```python
from build123d import *

# Parameters (mm, degrees)
SKETCH_1_W          = 30
SKETCH_1_H          = 16
EXTRUDE_1_DEPTH     = 2
EXTRUDE_2_DEPTH     = 1
SKETCH_3_R          = 2.5
EXTRUDE_3_DEPTH     = 15
SKETCH_4_W          = 7.5
SKETCH_4_H          = 13
SKETCH_5_R          = 3
CUT_EXTRUDE_1_DEPTH = 27.248809497


with BuildPart() as part:
    # 草圖1 → 填料-伸長1 (new body)
    with BuildSketch(Plane.XY):
        Rectangle(SKETCH_1_W, SKETCH_1_H)
    extrude(amount=EXTRUDE_1_DEPTH)

    # 草圖2 → 填料-伸長2 (add)
    with BuildSketch(Plane(origin=(0, 8, 0), x_dir=(1, 0, 0), z_dir=(0, 1, 0))):
        with BuildLine():
            Line((-15, 0), (15, 0))
            Line((15, 0), (15, 8))
            Line((15, 8), (12, 8))
            ThreePointArc((12, 8), (9.226499019, 8.839748528), (7.384615385, 11.076923077))
            ThreePointArc((7.384615385, 11.076923077), (0, 16), (-7.384615385, 11.076923077))
            ThreePointArc((-7.384615385, 11.076923077), (-9.226499019, 8.839748528), (-12, 8))
            Line((-12, 8), (-15, 8))
            Line((-15, 8), (-15, 0))
        make_face()
    extrude_2 = extrude(amount=-EXTRUDE_2_DEPTH)

    # 鏡射1: 填料-伸長2 across plane
    add(extrude_2.mirror(Plane.ZX))

    # 草圖3 → 填料-伸長3 (add)
    with BuildSketch(Plane(origin=(0, 8, 0), x_dir=(1, 0, 0), z_dir=(0, 1, 0))):
        with Locations(Location((0, 12, 0), (0, 0, 270))):
            Circle(SKETCH_3_R)
    extrude(amount=-EXTRUDE_3_DEPTH)

    # 草圖4 → 旋轉1 (revolve)
    with BuildSketch(Plane(origin=(0, 0, -12.5), x_dir=(-1, 0, 0), z_dir=(0, 0, -1))):
        with Locations((3.75, 0)):
            Rectangle(SKETCH_4_W, SKETCH_4_H)
    revolve(axis=Axis((0, 6.5, -12.5), (0, -1, 0)))

    # 草圖5 → 除料-伸長1 (cut, through all)
    with BuildSketch(Plane(origin=(0, 0, 0), x_dir=(-1, 0, 0), z_dir=(0, 0, -1))):
        with Locations((-11, 0)):
            Circle(SKETCH_5_R)
        with Locations((11, 0)):
            Circle(SKETCH_5_R)
    extrude(amount=-CUT_EXTRUDE_1_DEPTH, mode=Mode.SUBTRACT)


solid = part.part
```
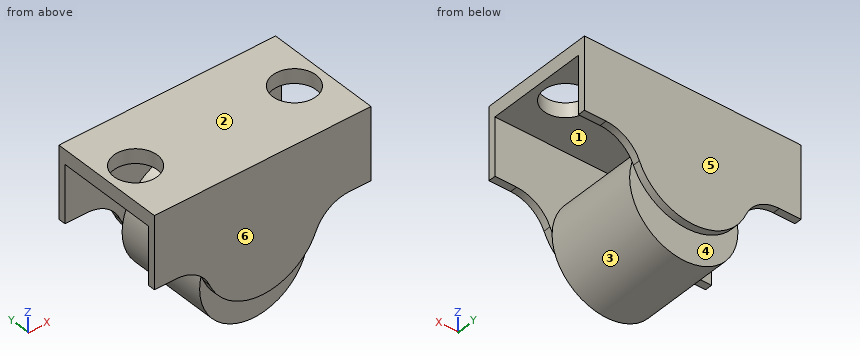
Can you work these out from the model? Positions are in its coordinate system, mm. Face numbers are marked on the shaded views. A direction names the side the tool comes from. Coordinates: 2 decimals unless noted, no trailing zeros. Loops run counter-clockwise (first coordinate to the right, second up) from the corner with the lowest first, then second, coordinate; pieces in that order, holes last.
1) Which directions (+Z, -Z, +X, -X, +Y, -Y) give clear straight access to the entire face, cutting with the end or side of a thin tool? Please do the marked faces 1, 2 and 3.
2) Imagine slicing it at B-B on x = 0. List the corners of the cut face in (y, z) for me, plus the area to 3 significant figures.
3) Imagine slicing it at C-C on y = 0. List the corners of the cut face in (x, z) for me.
4) Imagine slicing it at A-A on z = -0.75. List the corners of the cut face in (x, y) for me.
5) For pin 1 (4 mm diameter, centred on y = 3, z = -12, fed in from -X); pin 2 (5 mm diameter, centred on x = -3, y = 0.5, fed in from -Z); pin 3 (1.5 mm diameter, centred on y = -1, z = -3.5, fed in from +X); pin 4 (2 mm diameter, centred on y = -4.5, z = -17.5, fed in from +X), each with a flat end and sliding along its axis, tell me the tip position at first contact or that it passes through.
6) Imagine slicing it at D-D on z = -6.75. List the corners of the cut face in (x, y) for me.
7) Thinking about a two-plate mould opening in Y: for the marked faces 4, 5 and 6, which applies, pulls with the +Y half, pulls with the -Y half, needs draft (parallel to the pull), parting line crosses it, or undercut?
8) I need wall thicknesses on probe 1 along Y at (x, z) = (1.5, -8.5); probe 2 along X at (y, z) = (-0.5, 0.25); probe 3 along Y at (x, z) = (-11, 1.05). Which ranges of each line are inside material? Lowest first, please.
Completed:
1. face 1: +X, -X
1. face 2: +Z, +X, -X, +Y, -Y
1. face 3: none
2. outline: (-8, -16) - (-7, -16) - (-7, -14.5) - (-6.5, -14.5) - (-6.5, -20) - (6.5, -20) - (6.5, -14.5) - (7, -14.5) - (7, -16) - (8, -16) - (8, 2) - (-8, 2) - close; hole (-7, -9.5) - (-6.5, -9.5) - (-6.5, -5) - (6.5, -5) - (6.5, -9.5) - (7, -9.5) - (7, 0) - (-7, 0) - close
2. area: 264 mm2
3. outline: (-15, 0) - (-14, 0) - (-14, 2) - (-15, 2) - close; (-8, 0) - (8, 0) - (8, 2) - (-8, 2) - close; circle Ø15 at (0, -12.5); (14, 0) - (15, 0) - (15, 2) - (14, 2) - close
4. outline: (-15, -8) - (15, -8) - (15, -7) - (-15, -7) - close; (-15, 7) - (15, 7) - (15, 8) - (-15, 8) - close
5. pin 1: stops at x = -7.5
5. pin 2: stops at z = -19.98
5. pin 3: passes through
5. pin 4: stops at x = 6.34
6. outline: (-15, -8) - (15, -8) - (15, -7) - (-15, -7) - close; (-15, 7) - (15, 7) - (15, 8) - (-15, 8) - close; (-4.82, -6.5) - (4.82, -6.5) - (4.82, 6.5) - (-4.82, 6.5) - close
7. face 4: undercut
7. face 5: pulls with the +Y half
7. face 6: pulls with the -Y half
8. probe 1: y = -8 to -7, -6.5 to 6.5, 7 to 8
8. probe 2: x = -15 to -13.96, -8.04 to 8.04, 13.96 to 15
8. probe 3: y = -8 to -3, 3 to 8
